from build123d import *

# Parameters (mm, degrees)
SKETCH1_W                             = 73.025
SKETCH1_H                             = 6.35
EXTRUDE1_DEPTH                        = 182.5752
CUT_EXTRUDE1_DEPTH                    = 187.298654883
F_1_4_20_TAPPED_HOLE1_D               = 5.1054
F_1_8_0_125_DIAMETER_HOLE3_AT_2_COUNT = 2
F_1_8_0_125_DIAMETER_HOLE3_AT_2_PITCH = 12.7
F_1_8_0_125_DIAMETER_HOLE3_AT_3_COUNT = 2
F_1_8_0_125_DIAMETER_HOLE3_AT_3_PITCH = 276.2504
F_1_8_0_125_DIAMETER_HOLE3_AT_4_COUNT = 2
F_1_8_0_125_DIAMETER_HOLE3_AT_4_PITCH = 263.5504
CUT_EXTRUDE2_REACH                    = 188.299
SKETCH8_W                             = 50.8
SKETCH8_H                             = 9.525
CUT_EXTRUDE3_REACH                    = 188.299
SKETCH14_W                            = 50.8
SKETCH14_H                            = 1.5875
BOSS_EXTRUDE1_DEPTH                   = 6.35
FILLET1_R                             = 3.175
CUT_EXTRUDE4_REACH                    = 188.616
SKETCH18_W                            = 26.416
SKETCH18_H                            = 6.858
FILLET2_R                             = 0.79375
FILLET3_R                             = 9.525
F_9_32_0_28125_DIAMETER_HOLE2_D       = 7.14375
F_1_4_20_START                        = -4
F_1_4_20_TAPPED_HOLE2_OUTLINE_R       = 2.5527
F_1_4_20_TAPPED_HOLE2_DEPTH           = 8


with BuildPart() as part:
    # Sketch1 → Extrude1 (new, symmetric)
    with BuildSketch(Plane(origin=(0, 0, 0), x_dir=(0, 0, -1), z_dir=(1, 0, 0))):
        Rectangle(SKETCH1_W, SKETCH1_H)
    extrude(amount=EXTRUDE1_DEPTH, both=True)

    # Sketch2 → Cut-Extrude1 (cut, through all)
    with BuildSketch(Plane(origin=(0, 3.175, 0), x_dir=(-1, 0, 0), z_dir=(0, 1, 0))):
        with BuildLine():
            Line((100.01885, 7.9375), (100.01885, -36.5125))
            Line((100.01885, -36.5125), (52.39385, -36.5125))
            Line((52.39385, -36.5125), (52.39385, 7.9375))
            ThreePointArc((52.39385, 7.9375), (55.183657909, 14.672692091), (61.91885, 17.4625))
            Line((61.91885, 17.4625), (90.49385, 17.4625))
            ThreePointArc((90.49385, 17.4625), (97.229042091, 14.672692091), (100.01885, 7.9375))
        make_face()
    extrude(amount=-CUT_EXTRUDE1_DEPTH, mode=Mode.SUBTRACT)

    # 1/4-20 Tapped Hole1 (through all)
    with Locations(Plane(origin=(0, 3.175, 0), x_dir=(-1, 0, 0), z_dir=(0, 1, 0))):
        with Locations((146.05, -4.7625), (-17.4752, 8.73125), (-80.9752, -7.9375), (-146.05, -4.7625)):
            Hole(F_1_4_20_TAPPED_HOLE1_D / 2)

    # Sketch5 → 1/8 (0.125) Diameter Hole3 (revolve, cut)
    with BuildSketch(Plane(origin=(131.7752, 3.175, -33.3375), x_dir=(0, 0, 1), z_dir=(1, 0, 0))):
        Polygon((0, 0), (0, 6.35), (2.9765625, 6.35), (1.5875, 5.184438169), (1.5875, 1.165561831), (2.9765625, 0), align=None)
    f_1_8_0_125_diameter_hole3 = revolve(axis=Axis((131.7752, 9.525, -33.3375), (0, -1, 0)), mode=Mode.SUBTRACT)

    # 1/8 (0.125) Diameter Hole3 at 2: 1/8 (0.125) Diameter Hole3 ×2
    with Locations(*[(i * F_1_8_0_125_DIAMETER_HOLE3_AT_2_PITCH, 0, 0) for i in range(1, F_1_8_0_125_DIAMETER_HOLE3_AT_2_COUNT)]):
        add(f_1_8_0_125_diameter_hole3, mode=Mode.SUBTRACT)

    # 1/8 (0.125) Diameter Hole3 at 3: 1/8 (0.125) Diameter Hole3 ×2
    with Locations(*[(-i * F_1_8_0_125_DIAMETER_HOLE3_AT_3_PITCH, 0, 0) for i in range(1, F_1_8_0_125_DIAMETER_HOLE3_AT_3_COUNT)]):
        add(f_1_8_0_125_diameter_hole3, mode=Mode.SUBTRACT)

    # 1/8 (0.125) Diameter Hole3 at 4: 1/8 (0.125) Diameter Hole3 ×2
    with Locations(*[(-i * F_1_8_0_125_DIAMETER_HOLE3_AT_4_PITCH, 0, 0) for i in range(1, F_1_8_0_125_DIAMETER_HOLE3_AT_4_COUNT)]):
        add(f_1_8_0_125_diameter_hole3, mode=Mode.SUBTRACT)

    # Sketch8 → Cut-Extrude2 (cut, up to next)
    with BuildSketch(Plane(origin=(0, 3.175, 0), x_dir=(1, 0, 0), z_dir=(0, 1, 0)), mode=Mode.PRIVATE) as cut_extrude2_sk1:
        with Locations((-157.1752, -31.75)):
            Rectangle(SKETCH8_W, SKETCH8_H)
    cut_extrude2_tool1 = extrude(cut_extrude2_sk1.sketch, amount=-CUT_EXTRUDE2_REACH, mode=Mode.PRIVATE) & part.part
    # Sketch8 → Cut-Extrude2 (cut, up to next)
    with BuildSketch(Plane(origin=(0, 3.175, 0), x_dir=(1, 0, 0), z_dir=(0, 1, 0)), mode=Mode.PRIVATE) as cut_extrude2_sk2:
        with Locations((157.1752, -31.75)):
            Rectangle(SKETCH8_W, SKETCH8_H)
    cut_extrude2_tool2 = extrude(cut_extrude2_sk2.sketch, amount=-CUT_EXTRUDE2_REACH, mode=Mode.PRIVATE) & part.part
    add(cut_extrude2_tool1.solids().sort_by_distance((-157.1752, 3.175, 31.75))[0], mode=Mode.SUBTRACT)
    add(cut_extrude2_tool2.solids().sort_by_distance((157.1752, 3.175, 31.75))[0], mode=Mode.SUBTRACT)

    # Sketch13 → Cut-Extrude3 (cut, up to next)
    with BuildSketch(Plane(origin=(0, 3.175, 0), x_dir=(1, 0, 0), z_dir=(0, 1, 0)), mode=Mode.PRIVATE) as cut_extrude3_sk1:
        with BuildLine():
            Line((-52.39385, 36.5125), (77.8002, 36.5125))
            Line((77.8002, 36.5125), (77.8002, 30.1625))
            ThreePointArc((77.8002, 30.1625), (76.87026403, 27.91743597), (74.6252, 26.9875))
            Line((74.6252, 26.9875), (-52.39385, 26.9875))
            Line((-52.39385, 26.9875), (-52.39385, 36.5125))
        make_face()
    cut_extrude3_tool1 = extrude(cut_extrude3_sk1.sketch, amount=-CUT_EXTRUDE3_REACH, mode=Mode.PRIVATE) & part.part
    add(cut_extrude3_tool1.solids().sort_by_distance((12.590656, 3.175, -31.757083))[0], mode=Mode.SUBTRACT)

    # Sketch14 → Boss-Extrude1 (add)
    with BuildSketch(Plane(origin=(0, 3.175, 0), x_dir=(1, 0, 0), z_dir=(0, 1, 0))):
        with Locations((157.1752, 37.30625)):
            Rectangle(SKETCH14_W, SKETCH14_H)
        with Locations((-157.1752, 37.30625)):
            Rectangle(SKETCH14_W, SKETCH14_H)
    extrude(amount=-BOSS_EXTRUDE1_DEPTH)

    # Fillet1
    # the kernel refuses this fillet: 3.175 mm, written as the material it adds along each edge
    with BuildSketch(Plane(origin=(131.7752, 3.175, 26.9875), x_dir=(0, 0, 1), z_dir=(0, -1, 0)), Plane(origin=(-131.7752, 3.175, 26.9875), x_dir=(-1, 0, 0), z_dir=(0, -1, 0))) as fillet1_piece_1:
        with BuildLine():
            CenterArc((FILLET1_R, -FILLET1_R), FILLET1_R, 90, 90)
            Line((0, -FILLET1_R), (0, 0))
            Line((0, 0), (FILLET1_R, 0))
        make_face()
    extrude(amount=6.35)
    # the kernel refuses this fillet: 3.175 mm, written as the material it takes off along each edge
    with BuildSketch(Plane(origin=(182.5752, 11.1125, 26.9875), x_dir=(0, 0, -1), z_dir=(0, -1, 0)), Plane(origin=(77.8002, 11.1125, -36.5125), x_dir=(0, 0, 1), z_dir=(0, -1, 0)), Plane(origin=(182.5752, 11.1125, -38.1), x_dir=(-1, 0, 0), z_dir=(0, -1, 0)), Plane(origin=(-182.5752, 11.1125, -38.1), x_dir=(0, 0, 1), z_dir=(0, -1, 0)), Plane(origin=(-182.5752, 11.1125, 26.9875), x_dir=(1, 0, 0), z_dir=(0, -1, 0)), Plane(origin=(-131.7752, 11.1125, 36.5125), x_dir=(1, 0, 0), z_dir=(0, -1, 0))) as fillet1_2_piece_1:
        with BuildLine():
            CenterArc((FILLET1_R, -FILLET1_R), FILLET1_R, 90, 90)
            Line((0, -FILLET1_R), (0, 0))
            Line((0, 0), (FILLET1_R, 0))
        make_face()
    extrude(amount=22.225, mode=Mode.SUBTRACT)
    with BuildSketch(Plane(origin=(131.7752, 11.1125, 36.5125), x_dir=(-1, 0, 0), z_dir=(0, -1, 0))) as fillet1_2_piece_2:
        with BuildLine():
            CenterArc((FILLET1_R, FILLET1_R), FILLET1_R, 180, 90)
            Line((0, FILLET1_R), (0, 0))
            Line((0, 0), (FILLET1_R, 0))
        make_face()
    extrude(amount=22.225, mode=Mode.SUBTRACT)
    with BuildSketch(Plane(origin=(131.7752, 10.049076643, -38.1), x_dir=(0, 0, 1), z_dir=(0, -1, 0))) as fillet1_2_piece_3:
        with BuildLine():
            CenterArc((3.175, -2.749630657), FILLET1_R, 120, 60)
            Line((0, -2.749630657), (0, 0))
            Line((0, 0), (1.5875, 0))
        make_face()
    extrude(amount=20.098153285, mode=Mode.SUBTRACT)
    with BuildSketch(Plane(origin=(-131.7752, 10.049076643, -38.1), x_dir=(-1, 0, 0), z_dir=(0, -1, 0))) as fillet1_2_piece_4:
        with BuildLine():
            CenterArc((2.749630657, -3.175), FILLET1_R, 90, 60)
            Line((0, -1.5875), (0, 0))
            Line((0, 0), (2.749630657, 0))
        make_face()
    extrude(amount=20.098153285, mode=Mode.SUBTRACT)

    # Sketch18 → Cut-Extrude4 (cut, up to next)
    with BuildSketch(Plane(origin=(0, 3.175, 0), x_dir=(1, 0, 0), z_dir=(0, 1, 0)), mode=Mode.PRIVATE) as cut_extrude4_sk1:
        with Locations((0, -33.0835)):
            Rectangle(SKETCH18_W, SKETCH18_H)
    cut_extrude4_tool1 = extrude(cut_extrude4_sk1.sketch, amount=-CUT_EXTRUDE4_REACH, mode=Mode.PRIVATE) & part.part
    add(cut_extrude4_tool1.solids().sort_by_distance((0, 3.175, 33.0835))[0], mode=Mode.SUBTRACT)

    # Fillet2
    fillet2_edges = [part.edges().sort_by_distance(p)[0] for p in [
        (13.208, 0, 36.5125),
        (-13.208, 0, 36.5125),
    ]]
    fillet(fillet2_edges, radius=FILLET2_R)

    # Fillet3
    fillet3_edges = [part.edges().sort_by_distance(p)[0] for p in [
        (-52.39385, 0, -26.9875),
        (-100.01885, 0, -36.5125),
    ]]
    fillet(fillet3_edges, radius=FILLET3_R)

    # 9/32 (0.28125) Diameter Hole2 (through all)
    with Locations(Plane(origin=(0, 3.175, 0), x_dir=(1, 0, 0), z_dir=(0, 1, 0))):
        with Locations((-36.4998, -3.175), (-14.2748, -3.175)):
            Hole(F_9_32_0_28125_DIAMETER_HOLE2_D / 2)

    # 1/4-20 Tapped Hole2: read off the stored shape, not the designer's step
    # 1/4-20 Tapped Hole2 outline → 1/4-20 Tapped Hole2 (cut)
    with BuildSketch(Plane(origin=(0, 0, 0), x_dir=(1, 0, 0), z_dir=(0, 1, 0)).offset(F_1_4_20_START)):
        with Locations((-39.6875, 17.4625)):
            Circle(F_1_4_20_TAPPED_HOLE2_OUTLINE_R)
        with Locations((39.6875, 17.4625)):
            Circle(F_1_4_20_TAPPED_HOLE2_OUTLINE_R)
    extrude(amount=F_1_4_20_TAPPED_HOLE2_DEPTH, mode=Mode.SUBTRACT)


solid = part.part
Geometry check sheet. Reference: the model listing, model coordinates, mm. A direction names the side the tool comes from. Round coordinates to 2 decimals unless told otherwise and drop trailing zeros. Loops run counter-clockwise (first coordinate to the right, second up) from the corner with the lowest first, then second, coordinate; pieces in that order, holes last. Notation, with made-up numbers: (-3, 50) -> (24, 50) arc R25 cw to (24, 64) -> close; hole circle Ø9 at (14, 65). An arc over 180 degrees is marked (long way). Answer as a JSON object with one key per item and string values. Group by question number.
Item 1: Cross-section at B-B, the plane y = -0.25. Count the separate pieces of the cut face and the enclosed holes in it, plus the area to 3 significant figures.
Item 2: Release check for a two-part mould opening along X. For faces 4 (the face through (-121, 0, -36.512)), 5 (the face through (-3, -3.175, 0)), 6 (the face through (-182.575, 0, -5)) record: pulls with the +X half, pulls with the -X half, needs draft (parallel to the pull), parting line crosses it, or undercut.
Item 3: Depth check by flat-ended pin: pin 1 Ø3 at (y, z) = (1.5, 32) entering from +X; pin 2 Ø3 at (x, y) = (-3.5, 1.5) entering from +Z; pin 3 Ø1.9 at (x, y) = (-81, -0.5) entering from -Z. Enter the tip coordinate at first touch or a pass-through.
Item 4: Cross-section at C-C, the plane x = -23. Record the cut outline in (y, z) (1 decimal).
Item 5: Thickness scan on line 1 along X through (y, z) = (2.5, -17); line 2 along X through (y, z) = (-0.5, -18.5); line 3 along X through (y, z) = (-1.5, -14). Record the ranges inside material, lowest first.
Item 6: Set-up check for faces 1 (the face through (-49.5, 0, -24.3)), 2 (the face through (13.208, 0, 33)), 3 (the face through (-157, 0, 26.988)): record each of +Z, -Z, +X, -X, +Y, -Y from which the full face is reachable in a straight line by a thin tool's end or side.
Item 7: Cross-section at A-A, the plane x = 124.5. Record the cut outline in (y, z) (1 decimal), plus the area to 3 significant figures.
Determined:
{
 "1": {"separate pieces": "1", "enclosed holes": "12", "area": "21,600 mm²"},
 "2": {"face 4": "undercut", "face 5": "needs draft", "face 6": "pulls with the -X half"},
 "3": {"pin 1": "stops at x = 131.78", "pin 2": "stops at z = 29.65", "pin 3": "stops at z = 17.46"},
 "4": {"outline": "(-3.2, -27) -> (3.2, -27) -> (3.2, 36.5) -> (-3.2, 36.5) -> close"},
 "5": {"line 1": "x = -182.58 to -100.02, -52.39 to -42.2, -37.18 to 37.18, 42.2 to 182.58", "line 2": "x = -182.58 to -100.02, -52.34 to -42.02, -37.36 to 37.36, 42.02 to 182.58", "line 3": "x = -182.58 to -100.02, -52.39 to 182.58"},
 "6": {"face 1": "-Z, +Y, -Y", "face 2": "+Z, +Y, -Y", "face 3": "+Z, -X, +Y, -Y"},
 "7": {"outline": "(-3.2, -36.5) -> (3.2, -36.5) -> (3.2, 36.5) -> (-3.2, 36.5) -> close", "area": "464 mm²"}
}
